Input: part model. Units: mm. Frame: model coordinates. A direction names the side the tool comes from. Give positions to 0.01 mm unless a question says otherwise; leave off trailing zeros. Order: outer loops, then holes, each group sorted by start corner. A loop starts at its lowest first (then second) coordinate and runs counter-clockwise, first axis right, second up. Notation, with made-up numbers: (16.25, 0) -> (71.25, 0) arc R27 ccw to (71.25, 34) -> close; hole circle Ø6 at (35.5, -0.5). An arc over 180 degrees is marked (long way). Use a Markdown table: item, result. Add a question column.
from build123d import *

# Parameters (mm, degrees)
EXTRUDE_1_DEPTH      = 14
CUT_EXTRUDE_1_DEPTH  = 44
SKETCH_3_W           = 6.2
SKETCH_3_H           = 6.2
CUT_EXTRUDE_2_DEPTH  = 4
SKETCH_4_R           = 4
CUT_EXTRUDE_3_DEPTH  = 5
SKETCH_5_R           = 2.6
CUT_EXTRUDE_4_DEPTH  = 5
EXTRUDE_2_DEPTH      = 44
SKETCH_8_W           = 5
SKETCH_8_H           = 5
EXTRUDE_4_DEPTH      = 15
SKETCH_9_W           = 35
SKETCH_9_H           = 5
EXTRUDE_5_DEPTH      = 7
CUT_EXTRUDE_6_DEPTH  = 10
CUT_EXTRUDE_START    = -30
SKETCH_14_R          = 1.55
CUT_EXTRUDE_7_DEPTH  = 30
SKETCH_15_R          = 3
CUT_EXTRUDE_8_DEPTH  = 2
CUT_EXTRUDE_START_2  = -2
SKETCH_16_R          = 3
CUT_EXTRUDE_9_DEPTH  = 2
SKETCH_17_W          = 35
SKETCH_17_H          = 7
CUT_EXTRUDE_10_DEPTH = 10
SKETCH_18_W          = 35
SKETCH_18_H          = 7
CUT_EXTRUDE_11_DEPTH = 20
SKETCH_19_R          = 5
CUT_EXTRUDE_12_DEPTH = 7


with BuildPart() as part:
    # 草图1 → 凸台-拉伸1 (new body)
    with BuildSketch(Plane.XY):
        Polygon((-15, 22), (-15, -22), (15, -22), (15, 22), (0, 22), align=None)
    extrude(amount=EXTRUDE_1_DEPTH)

    # 草图2 → 切除-拉伸1 (cut)
    with BuildSketch(Plane(origin=(0, 22, 0), x_dir=(1, 0, 0), z_dir=(0, 1, 0))):
        Polygon((-15, 0), (-15, -14), (-10, -4), (-3.1, -4), (-3.1, 0), align=None)
        Polygon((3.1, -4), (10, -4), (15, -14), (15, 0), (3.1, 0), align=None)
    extrude(amount=-CUT_EXTRUDE_1_DEPTH, mode=Mode.SUBTRACT)

    # 草图3 → 切除-拉伸2 (cut)
    with BuildSketch(Plane(origin=(0, 0, 0), x_dir=(-1, 0, 0), z_dir=(0, 0, -1))):
        Rectangle(SKETCH_3_W, SKETCH_3_H)
    extrude(amount=-CUT_EXTRUDE_2_DEPTH, mode=Mode.SUBTRACT)

    # 草图4 → 切除-拉伸3 (cut)
    with BuildSketch(Plane.XY.offset(14)):
        Circle(SKETCH_4_R)
    extrude(amount=-CUT_EXTRUDE_3_DEPTH, mode=Mode.SUBTRACT)

    # 草图5 → 切除-拉伸4 (cut)
    with BuildSketch(Plane.XY.offset(9)):
        Circle(SKETCH_5_R)
    extrude(amount=-CUT_EXTRUDE_4_DEPTH, mode=Mode.SUBTRACT)

    # 草图7 → 凸台-拉伸2 (add)
    with BuildSketch(Plane.XZ.offset(22)):
        Polygon((15, 14), (20, 14), (20, 9), (10, 4), (10, 14), align=None)
    extrude(amount=-EXTRUDE_2_DEPTH)

    # 草图8 → 凸台-拉伸4 (add)
    with BuildSketch(Plane.XY.offset(14)):
        with Locations((-12.5, -12.5)):
            Rectangle(SKETCH_8_W, SKETCH_8_H)
        Polygon((-10, -10), (-10, -15), (10, -15), (10, -10), (0, -10), align=None)
        Polygon((-10, 0), (-10, 10), (-15, 10), (-15, -10), (-10, -10), align=None)
        with Locations((-12.5, 12.5)):
            Rectangle(SKETCH_8_W, SKETCH_8_H)
        Polygon((-10, 15), (10, 15), (10, 10), (0, 10), (-10, 10), align=None)
        with Locations((12.5, 12.5)):
            Rectangle(SKETCH_8_W, SKETCH_8_H)
        Polygon((15, 10), (15, -10), (10, -10), (10, 0), (10, 10), align=None)
        with Locations((12.5, -12.5)):
            Rectangle(SKETCH_8_W, SKETCH_8_H)
        with Locations((17.5, -12.5)):
            Rectangle(SKETCH_8_W, SKETCH_8_H)
        with Locations((17.5, 12.5)):
            Rectangle(SKETCH_8_W, SKETCH_8_H)
    extrude(amount=EXTRUDE_4_DEPTH)

    # 草图9 → 凸台-拉伸5 (add)
    with BuildSketch(Plane(origin=(0, 15, 0), x_dir=(1, 0, 0), z_dir=(0, 1, 0))):
        with Locations((2.5, -26.5)):
            Rectangle(SKETCH_9_W, SKETCH_9_H)
    extrude(amount=EXTRUDE_5_DEPTH)

    # 草图13 → 切除-拉伸6 (cut)
    with BuildSketch(Plane(origin=(-10, 0, 0), x_dir=(0, 0, -1), z_dir=(1, 0, 0))):
        with BuildLine():
            ThreePointArc((-19.95, 0), (-20.806818927, 1.386362146), (-22.43, 1.24))
            Line((-22.43, 1.24), (-20.57, -1.24))
            ThreePointArc((-20.57, -1.24), (-20.113637854, -0.693181073), (-19.95, 0))
        make_face()
        with BuildLine():
            Line((-20.57, -1.24), (-22.43, 1.24))
            ThreePointArc((-22.43, 1.24), (-22.74, -0.93), (-20.57, -1.24))
        make_face()
    extrude(amount=-CUT_EXTRUDE_6_DEPTH, mode=Mode.SUBTRACT)

    # 草图14 → 切除-拉伸7 (cut)
    with BuildSketch(Plane.ZY.offset(15).offset(CUT_EXTRUDE_START)):
        with Locations(Location((21.5, 0, 0), (0, 0, 180))):
            Circle(SKETCH_14_R)
    extrude(amount=CUT_EXTRUDE_7_DEPTH, mode=Mode.SUBTRACT)

    # 草图15 → 切除-拉伸8 (cut)
    with BuildSketch(Plane(origin=(15, 0, 0), x_dir=(0, 0, -1), z_dir=(1, 0, 0))):
        with Locations((-21.5, 0)):
            Circle(SKETCH_15_R)
    extrude(amount=-CUT_EXTRUDE_8_DEPTH, mode=Mode.SUBTRACT)

    # 草图16 → 切除-拉伸9 (cut)
    with BuildSketch(Plane.ZY.offset(15).offset(CUT_EXTRUDE_START_2)):
        with Locations(Location((21.5, 0, 0), (0, 0, 180))):
            Circle(SKETCH_16_R)
    extrude(amount=CUT_EXTRUDE_9_DEPTH, mode=Mode.SUBTRACT)

    # 草图17 → 切除-拉伸10 (cut)
    with BuildSketch(Plane.XY.offset(29)):
        with Locations((2.5, 18.5)):
            Rectangle(SKETCH_17_W, SKETCH_17_H)
    extrude(amount=-CUT_EXTRUDE_10_DEPTH, mode=Mode.SUBTRACT)

    # 草图18 → 切除-拉伸11 (cut)
    with BuildSketch(Plane.XY.offset(14)):
        with Locations((2.5, 18.5)):
            Rectangle(SKETCH_18_W, SKETCH_18_H)
        with Locations((2.5, -18.5)):
            Rectangle(SKETCH_18_W, SKETCH_18_H)
    extrude(amount=-CUT_EXTRUDE_11_DEPTH, mode=Mode.SUBTRACT)

    # 草图19 → 切除-拉伸12 (cut)
    with BuildSketch(Plane.XY.offset(14)):
        Circle(SKETCH_19_R)
    extrude(amount=-CUT_EXTRUDE_12_DEPTH, mode=Mode.SUBTRACT)


solid = part.part
Q1. Section query B-B (x = 0). Return loops of the section in (y, z), plus the area to 3 significant figures.
Q2. Draft query along Y for faces 6 (the cylindrical face through (-14, -0.1, 24.5)), 7 (the flat face through (2, -15, 18)), 8 (the flat face through (0, 9, 0)). Return one class per face: +Y half, -Y half, draft (parallel to the pull), parting line (faces both ways), or undercut.
Q3. Section query C-C (y = 12). Return loops of the section in (x, z), plus the area to 3 significant figures.
Q4. Access query for faces 1 (the flat face through (13, -1, 20)), 2 (the flat face through (0, 3.1, 2)), 3 (the flat face through (15, 0, 18)), 4 (the flat face through (-13, 1, 20)), 5 (the flat face through (2, -5, 14)). Directions: +Z, -Z, +X, -X, +Y, -Y. A direction counts if a zero-diameter tool reaches every point of the face in a straight line with its end or side. Return the directions, or none.
Q5. Section query A-A (z = 21.5). Return loops of the section in (x, y), plus the area to 3 significant figures.
Q6. First-contact query: pin 1 (8 mm diameter, centred on x = 1, y = 1, fed in from +Z); pin 2 (6.5 mm diameter, centred on y = 0.5, z = 21, fed in from -X); pin 3 (4.5 mm diameter, centred on y = 7.5, z = 1.5, fed in from -X); pin 4 (3.5 mm diameter, centred on y = 0, z = 21.5, fed in from -X). Flat tips, straight axial feed; report the tip coordinate or a pass-through.
Q7. Ray query, line 1 (Y direction, x = 0, z = 9); line 2 (Y direction, x = 0, z = 5.6); line 3 (X direction, y = -5, z = 15.75). Return the intervals inside material, ascending.
Q8. Section query D-D (z = 15.75). Return loops of the section in (x, y), plus the area to 3 significant figures.
Solution:
| question | item | result |
|---|---|---|
| 1 | outline | (-15, 0) -> (-3.1, 0) -> (-3.1, 4) -> (-2.6, 4) -> (-2.6, 7) -> (-5, 7) -> (-5, 14) -> (-10, 14) -> (-10, 29) -> (-15, 29) -> close; (2.6, 4) -> (3.1, 4) -> (3.1, 0) -> (15, 0) -> (15, 29) -> (10, 29) -> (10, 14) -> (5, 14) -> (5, 7) -> (2.6, 7) -> close |
| 1 | area | 460 mm² |
| 2 | face 6 | undercut |
| 2 | face 7 | -Y half |
| 2 | face 8 | draft |
| 3 | outline | (-15, 14) -> (-10, 4) -> (-3.1, 4) -> (-3.1, 0) -> (3.1, 0) -> (3.1, 4) -> (10, 4) -> (20, 9) -> (20, 29) -> (-15, 29) -> close |
| 3 | area | 850 mm² |
| 4 | face 1 | +X |
| 4 | face 2 | -Z, +X, -X |
| 4 | face 3 | +Z, +X |
| 4 | face 4 | -X |
| 4 | face 5 | +Z |
| 5 | outline | (-15, -15) -> (20, -15) -> (20, -10) -> (15, -10) -> (15, -3) -> (13, -3) -> (13, -1.55) -> (10, -1.55) -> (10, -10) -> (-10, -10) -> (-10, -1.55) -> (-13, -1.55) -> (-13, -3) -> (-15, -3) -> close; (-15, 3) -> (-13, 3) -> (-13, 1.55) -> (-10, 1.55) -> (-10, 10) -> (10, 10) -> (10, 1.55) -> (13, 1.55) -> (13, 3) -> (15, 3) -> (15, 10) -> (20, 10) -> (20, 15) -> (-15, 15) -> close |
| 5 | area | 507 mm² |
| 6 | pin 1 | stops at z = 14 |
| 6 | pin 2 | stops at x = -15 |
| 6 | pin 3 | stops at x = -3.1 |
| 6 | pin 4 | stops at x = -13 |
| 7 | line 1 | y = -15 to -5, 5 to 15 |
| 7 | line 2 | y = -15 to -2.6, 2.6 to 15 |
| 7 | line 3 | x = -15 to -10, 10 to 15 |
| 8 | outline | (-15, -15) -> (20, -15) -> (20, -10) -> (15, -10) -> (15, 10) -> (20, 10) -> (20, 15) -> (-15, 15) -> close; hole (-10, -10) -> (10, -10) -> (10, 10) -> (-10, 10) -> close |
| 8 | area | 550 mm² |
